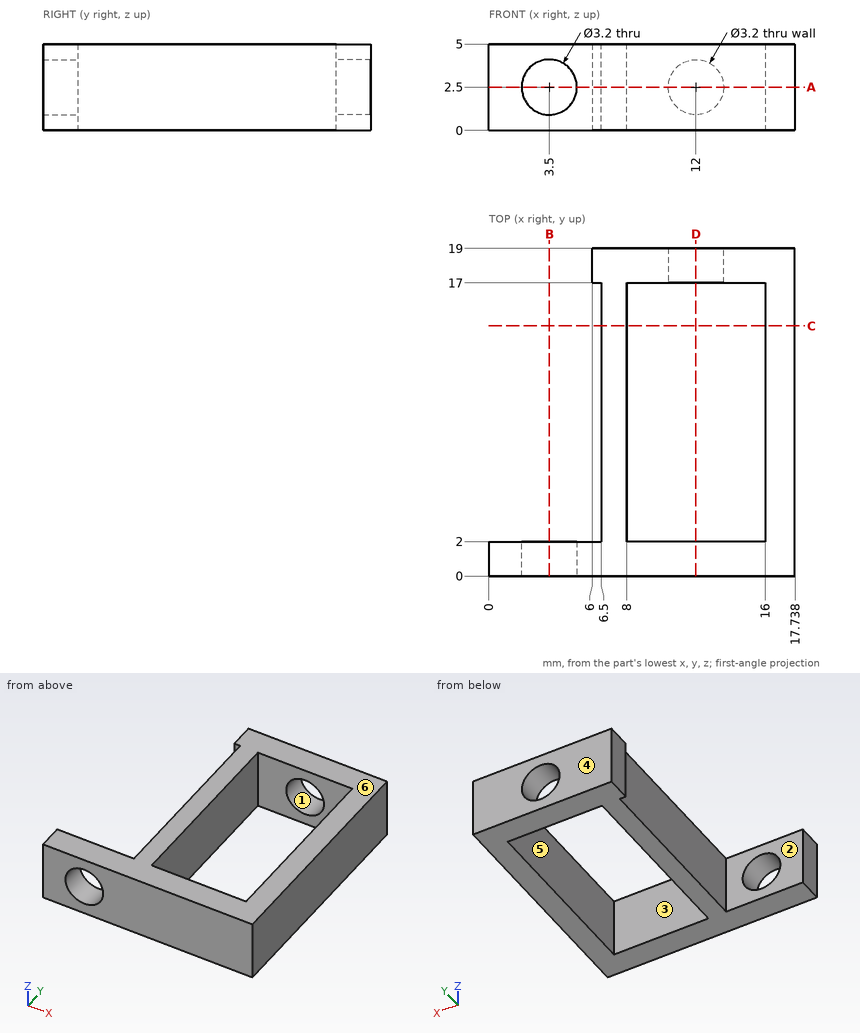
Design review of the part shown in the three views and the two pictorial views. Dimensions are in mm from the part's minimum x, y and z. A direction names the side the tool comes from. Coordinates: 2 decimals unless noted, no trailing zeros. Loops run counter-clockwise (first coordinate to the right, second up) from the corner with the lowest first, then second, coordinate; pieces in that order, holes last.
(1) Insertion check: P1, Ø2, axis at y = 18, z = 2.5, coming from the -X side; P2, Ø2, axis at y = 4, z = 4.5, coming from the -X side. Each pin has a flat end and moves straight along its axis. Give the tip position at first contact, or say it passes through.
Determined:
P1: stops at x = 6
P2: stops at x = 6.5
(2) Consider section C-C, the plane y = 14.5. Give the boundary of the cut face in (x, z), plus the area to 3 significant figures.
Determined:
outline: (6.5, 0) - (8, 0) - (8, 5) - (6.5, 5) - close; (16, 0) - (17.74, 0) - (17.74, 5) - (16, 5) - close
area: 16.2 mm2
(3) Consider section D-D, the plane x = 12. Give the boundary of the cut face in (y, z), plus the area to 3 significant figures.
Determined:
outline: (0, 0) - (2, 0) - (2, 5) - (0, 5) - close; (17, 0) - (19, 0) - (19, 0.9) - (17, 0.9) - close; (17, 4.1) - (19, 4.1) - (19, 5) - (17, 5) - close
area: 13.6 mm2
(4) Tool access review of the marked faces 1, 2 and 3: name each direction out of +Z, -Z, +X, -X, +Y, -Y from which nothing blocks a thin tool from reaching the whole face with its end or side.
Determined:
face 1: +Y
face 2: +Z, -Z, -X
face 3: +Z, -Z
(5) Consider section B-B, the plane x = 3.5. Give the boundary of the cut face in (y, z).
Determined:
outline: (0, 0) - (2, 0) - (2, 0.9) - (0, 0.9) - close; (0, 4.1) - (2, 4.1) - (2, 5) - (0, 5) - close
(6) Draft analysis for pull direction Y (two halves, no side actions). For the marked faces 4, 5 and 6, state which applies: +Y half, -Y half, draft (parallel to the pull), parting line (faces both ways), or undercut.
Determined:
face 4: +Y half
face 5: undercut
face 6: draft
(7) Consider section A-A, the plane z = 2.5. Give the boundary of the cut face in (x, y).
Determined:
outline: (0, 0) - (1.9, 0) - (1.9, 2) - (0, 2) - close; (5.1, 0) - (17.74, 0) - (17.74, 19) - (13.6, 19) - (13.6, 17) - (16, 17) - (16, 2) - (8, 2) - (8, 17) - (10.4, 17) - (10.4, 19) - (6, 19) - (6, 17) - (6.5, 17) - (6.5, 2) - (5.1, 2) - close
(8) Wall thickness on L1, parallel to Y at x = 14.5, z = 3.75; L2, parallel to Z at x = 3.5, y = 0.95; L3, parallel to X at y = 15.5, z = 1.45: over which ranges is each line inside the solid? List them lowest first.
Determined:
L1: y = 0 to 2, 17 to 19
L2: z = 0 to 0.9, 4.1 to 5
L3: x = 6.5 to 8, 16 to 17.74
